Work out the finished part from the listing and answer in its coordinate system (mm). A direction names the side the tool comes from. Round coordinates to 2 decimals unless told otherwise and drop trailing zeros. Order: outer loops, then holes, each group sorted by start corner. A loop starts at its lowest first (then second) coordinate and runs counter-clockwise, first axis right, second up. Notation, with made-up numbers: (0.25, 72.5) - (56.25, 72.5) arc R28 ccw to (56.25, 102.5) - close; hole circle Ø10 at (-38.75, 58.25). An arc over 180 degrees is marked (long way). Use one line per item in the form item = value. Start each with the question number.
Q1. Given P1, Ø2, axis at x = -0.5, y = -2, coming from the +Z side; P2, Ø1.5, axis at y = -2.5, z = -9, coming from the -X side, each flat-ended and moving along its own axis, determine where each tip first touches the part or whether it passes through.
Q2. For a pull along X with two mould halves and no side action, classify faces 4 (the flat face through (2.5, -2, 1)), 5 (the flat face through (-2.5, -2, 1)), 6 (the flat face through (0, -2, 31.118)) as +X half, -X half, draft (parallel to the pull), parting line (faces both ways), or undercut.
Q3. The part is cut by section B-B on x = -14. Determine the outline of the cut face in (y, z), plus the area to 3 significant figures.
Q4. The part is cut by section C-C on y = -2.6. Determine the outline of the cut face in (x, z), plus the area to 3 significant figures.
Q5. Find the intervals of material crossed by line 1 (Z direction, x = -4, y = -3.5); line 2 (X direction, y = -0.95, z = 32); line 3 (X direction, y = -4.7, z = 7), in increasing order. Write a range as [from, to].
Q6. Which of the six approach directions +Z, -Z, +X, -X, +Y, -Y give full straight-line access (tool end or side, diameter ignored) to faces 1 (the flat face through (-30, -2, 46)), 2 (the flat face through (-14, -2, -23.882)), 3 (the flat face through (-25, -2, -26))?
Q7. The part is cut by section D-D on z = -3.5. Determine the outline of the cut face in (x, y).
Q8. The part is cut by section A-A on z = 40.5. Determine the outline of the cut face in (x, y).
from build123d import *

# Parameters (mm, degrees)
F0_W     = 5
F0_H     = 50
F0_H_2   = 30
F1_DEPTH = 5


# Not quite as in the source:
# - a feature of the source that left no trace in its solid (it failed there, or was rolled back) is left out


with BuildPart() as f1:
    # F0 (on Front) → F1 (new body)
    with BuildSketch(Plane.XZ):
        Polygon((-35, 26.1184218031), (-2.5, 26.1184218031), (2.5, 26.1184218031), (35, 26.1184218031), (35, 31.1184218031), (30, 31.1184218031), (-30, 31.1184218031), (-35, 31.1184218031), align=None)
        with Locations((0, 1.1184218031)):
            Rectangle(F0_W, F0_H)
        Polygon((2.5, -23.8815781969), (-2.5, -23.8815781969), (-25, -23.8815781969), (-25, -28.8815781969), (25, -28.8815781969), (25, -23.8815781969), align=None)
        with Locations((-32.5, 46.1184218031)):
            Rectangle(F0_W, F0_H_2)
        with Locations((32.5, 46.1184218031)):
            Rectangle(F0_W, F0_H_2)
    extrude(amount=F1_DEPTH)


solid = f1.part
Found:
q1.P1 = 31.12
q1.P2 = -2.5
q2.face_4 = +X half
q2.face_5 = -X half
q2.face_6 = undercut
q3.outline = (-5, -28.88) - (0, -28.88) - (0, -23.88) - (-5, -23.88) - close; (-5, 26.12) - (0, 26.12) - (0, 31.12) - (-5, 31.12) - close
q3.area = 50.0 mm²
q4.outline = (-35, 26.12) - (-2.5, 26.12) - (-2.5, -23.88) - (-25, -23.88) - (-25, -28.88) - (25, -28.88) - (25, -23.88) - (2.5, -23.88) - (2.5, 26.12) - (35, 26.12) - (35, 61.12) - (30, 61.12) - (30, 31.12) - (-30, 31.12) - (-30, 61.12) - (-35, 61.12) - close
q4.area = 1,150 mm²
q5.line_1 = [-28.88, -23.88], [26.12, 31.12]
q5.line_2 = [-35, -30], [30, 35]
q5.line_3 = [-2.5, 2.5]
q6.face_1 = +Z, +Y, -Y
q6.face_2 = -X, +Y, -Y
q6.face_3 = -Z, -X, +Y, -Y
q7.outline = (-2.5, -5) - (2.5, -5) - (2.5, 0) - (-2.5, 0) - close
q8.outline = (-35, -5) - (-30, -5) - (-30, 0) - (-35, 0) - close; (30, -5) - (35, -5) - (35, 0) - (30, 0) - close
